Build history of the part. All positions in model axes, mm. Face numbers are marked on the shaded views. A direction names the side the tool comes from. Round coordinates to 2 decimals unless told otherwise and drop trailing zeros. Write each loop counter-clockwise with the first axis right and the second up, starting at its lowest first coordinate (ties: lowest second). Pieces come first, ordered by that corner, then holes. Notation, with made-up numbers: (55.25, -20.75) -> (96.25, -20.75) arc R16 cw to (96.25, -11.75) -> close; hole circle Ø6 at (4.5, 54). An arc over 180 degrees is marked (long way). Answer as CSV lines item,"result".
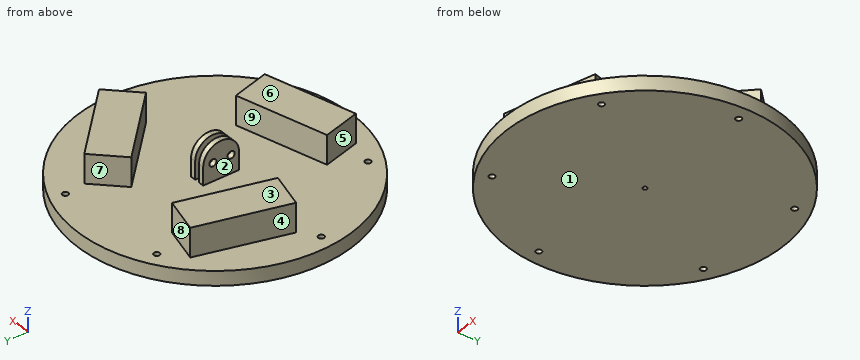
from build123d import *

# Parameters (mm, degrees)
SKETCH2_R           = 38.1
BOSS_EXTRUDE1_DEPTH = 4
SKETCH3_R           = 0.8
CUT_EXTRUDE1_DEPTH  = 6
SKETCH4_R           = 0.6
CUT_EXTRUDE2_DEPTH  = 6
SKETCH5_W           = 1.5
SKETCH5_H           = 10
BOSS_EXTRUDE2_DEPTH = 10
CUT_EXTRUDE3_DEPTH  = 58.198776211
SKETCH7_R           = 1
CUT_EXTRUDE4_DEPTH  = 58.198776211
BOSS_EXTRUDE3_DEPTH = 8
SKETCH10_R          = 0.8
CUT_EXTRUDE5_DEPTH  = 55.801642311


with BuildPart() as part:
    # Sketch2 → Boss-Extrude1 (new body)
    with BuildSketch(Plane.XY):
        Circle(SKETCH2_R)
    extrude(amount=BOSS_EXTRUDE1_DEPTH)

    # Sketch3 → Cut-Extrude1 (cut)
    with BuildSketch(Plane.XY.offset(4)):
        with Locations((34.1, -0.085721815)):
            Circle(SKETCH3_R)
        with Locations((-17.05, -29.617188084)):
            Circle(SKETCH3_R)
        with Locations((-17.05, 29.445744454)):
            Circle(SKETCH3_R)
    extrude(amount=-CUT_EXTRUDE1_DEPTH, mode=Mode.SUBTRACT)

    # Sketch4 → Cut-Extrude2 (cut)
    with BuildSketch(Plane.XY.offset(4)):
        Circle(SKETCH4_R)
    extrude(amount=-CUT_EXTRUDE2_DEPTH, mode=Mode.SUBTRACT)

    # Sketch5 → Boss-Extrude2 (add)
    with BuildSketch(Plane.XY.offset(4)):
        with Locations((1.45, 0)):
            Rectangle(SKETCH5_W, SKETCH5_H)
        with Locations((-1.45, 0)):
            Rectangle(SKETCH5_W, SKETCH5_H)
    extrude(amount=BOSS_EXTRUDE2_DEPTH)

    # Sketch6 → Cut-Extrude3 (cut, through all)
    with BuildSketch(Plane(origin=(2.2, 0, 0), x_dir=(0, 0, -1), z_dir=(1, 0, 0))):
        with BuildLine():
            ThreePointArc((-14, 0), (-12.535533906, 3.535533906), (-9, 5))
            Line((-9, 5), (-14, 5))
            Line((-14, 5), (-14, 0))
        make_face()
        with BuildLine():
            ThreePointArc((-9, -5), (-12.535533906, -3.535533906), (-14, 0))
            Line((-14, 0), (-14, -5))
            Line((-14, -5), (-9, -5))
        make_face()
    extrude(amount=-CUT_EXTRUDE3_DEPTH, mode=Mode.SUBTRACT)

    # Sketch7 → Cut-Extrude4 (cut, through all)
    with BuildSketch(Plane(origin=(2.2, 0, 0), x_dir=(0, 0, -1), z_dir=(1, 0, 0))):
        with Locations(Location((-9, 2.3, 0), (0, 0, 90))):
            Circle(SKETCH7_R)
        with Locations(Location((-9, -2.8, 0), (0, 0, 90))):
            Circle(SKETCH7_R)
    extrude(amount=-CUT_EXTRUDE4_DEPTH, mode=Mode.SUBTRACT)

    # Sketch8 → Boss-Extrude3 (add)
    with BuildSketch(Plane.XY.offset(4)):
        Polygon((25.028792455, 0), (32.453413657, 7.424621202), (14.492901415, 25.385133445), (7.068280213, 17.960512242), align=None)
        Polygon((12.02011976, -15.101566346), (14.737719734, -25.243787522), (-9.796796254, -31.817791268), (-12.514396227, -21.675570092), align=None)
        Polygon((-19.088399973, -2.858945896), (-29.230621149, -0.141345922), (-22.656617403, 24.393170065), (-12.514396227, 21.675570092), align=None)
    extrude(amount=BOSS_EXTRUDE3_DEPTH)

    # Sketch10 → Cut-Extrude5 (cut, through all)
    with BuildSketch(Plane.XY.offset(4)):
        with Locations((13.886765868, 31.144304997)):
            Circle(SKETCH10_R)
        with Locations((20.028376376, -27.598444517)):
            Circle(SKETCH10_R)
        with Locations((-33.915142244, -3.54586048)):
            Circle(SKETCH10_R)
    extrude(amount=-CUT_EXTRUDE5_DEPTH, mode=Mode.SUBTRACT)


solid = part.part
1. Cut at A-A, the plane z = 5. Write the cut outline in (x, y), then the cut area to 3 significant figures.
Results found:
outline,"(-29.23, -0.14) -> (-19.09, -2.86) -> (-12.51, 21.68) -> (-22.66, 24.39) -> close; (-12.51, -21.68) -> (-9.8, -31.82) -> (14.74, -25.24) -> (12.02, -15.1) -> close; (-2.2, -5) -> (-0.7, -5) -> (-0.7, 5) -> (-2.2, 5) -> close; (0.7, -5) -> (2.2, -5) -> (2.2, 5) -> (0.7, 5) -> close; (7.07, 17.96) -> (25.03, 0) -> (32.45, 7.42) -> (14.49, 25.39) -> close"
area,"830 mm2"
2. Mould opens along X. For the marked faces 6, 7, 8 and 9 say: +X half, -X half, draft (parallel to the pull), parting line (faces both ways), or undercut.
Results found:
face 6,"draft"
face 7,"undercut"
face 8,"undercut"
face 9,"-X half"
3. Drop flat-ended pins along their axis: pin 1 Ø2.5 at (y, z) = (-2.8, 9) entering from +X; pin 2 Ø1 at (x, z) = (0.5, 11) entering from -Y; pin 3 Ø4 at (x, y) = (-22, -18.5) entering from -Z; pin 4 Ø4 at (y, z) = (-30, 5.5) entering from -X. Give the stop position or say it passes through.
Results found:
pin 1,"stops at x = 2.2"
pin 2,"stops at y = -29.19"
pin 3,"stops at z = 0"
pin 4,"stops at x = -25.08"
4. Which spindle directions (+Z, -Z, +X, -X, +Y, -Y) get a long thin tool onto all of the face, cutting with end or side? Do the marked faces 1, 2, 3, 4 and 5. Say none if no direction does.
Results found:
face 1,"-Z, +X, -X, +Y, -Y"
face 2,"+Z, +Y"
face 3,"+Z, -X, +Y, -Y"
face 4,"+Z, -X, +Y"
face 5,"+Z, -X, -Y"
5. Cut at B-B, the plane x = 9. Write the cut outline in (y, z).
Results found:
outline,"(-37.02, 0) -> (37.02, 0) -> (37.02, 4) -> (19.89, 4) -> (19.89, 12) -> (16.03, 12) -> (16.03, 4) -> (-15.91, 4) -> (-15.91, 12) -> (-26.78, 12) -> (-26.78, 4) -> (-37.02, 4) -> close"
6. Probe line 1 along X through (y, z) = (1, 8.5); line 2 along Y through (x, z) = (-17.05, 1.5); line 3 along Z through (x, y) = (-26, -2). List the from-to ranges inside material, lowest first.
Results found:
line 1,"x = -28.92 to -18.05, -2.2 to -0.7, 0.7 to 2.2, 24.03 to 26.03"
line 2,"y = -34.07 to -30.42, -28.82 to 28.65, 30.25 to 34.07"
line 3,"z = 0 to 4"
7. Cut at C-C, the plane y = 13. Write the cut outline in (x, z), then the cut area to 3 significant figures.
Results found:
outline,"(-35.81, 0) -> (35.81, 0) -> (35.81, 4) -> (26.88, 4) -> (26.88, 12) -> (12.03, 12) -> (12.03, 4) -> (-14.84, 4) -> (-14.84, 12) -> (-25.71, 12) -> (-25.71, 4) -> (-35.81, 4) -> close"
area,"492 mm2"
